Can you work these out from the model? Positions are in its coordinate system, mm. A direction names the side the tool comes from. Round coordinates to 2 decimals unless told otherwise and drop trailing zeros. One line per item, written item: value. Start each with the question number.
(1) Thinking about a two-plate mould opening in X: for faces 1 (the face through (162.11, 20.5, 55.06)), 2 (the face through (149, 21, 77)), which applies, +X half, -X half, draft (parallel to the pull), parting line (faces both ways), or undercut?
(2) I'm going to push flat-ended pins straight in: pin 1 Ø4 at (y, z) = (14.5, 18) entering from -X; pin 2 Ø1 at (y, z) = (22, 49) entering from +X; pin 3 Ø8 at (y, z) = (23, 10.5) entering from +X. Where does each tip first touch, or does it pass through?
(3) If I drill on L1, parallel to Z at x = 140, y = 22.75; L2, parallel to X at y = 14.75, z = 41; L3, parallel to Z at x = 165, y = 20, over which ranges is the centre line in solid material (lowest first)? Write a range as from..to.
(4) I want a section at A-A on z = 32.5. Give the number of separate pieces and of enclosed holes in the cut face, plus the area to 3 significant figures.
(5) On a 3-axis mill with a long thin cutter (end or side, diameter ignored), from which of +Z, -Z, +X, -X, +Y, -Y can I reach the whole of each face in a straight line? I mean faces 3 (the face through (202.885, 11.105, 37.961)), 4 (the face through (153.56, 21.07, 69.94)), 5 (the face through (195.747, 17.752, 38.969)). Say none if no direction works.
Autodesk Inventor part; units mm, degrees
ref_plane "YZ Plane" through (0, 0, 0) normal (1, 0, 0) x (0, 1, 0)
ref_plane "XZ Plane" through (0, 0, 0) normal (0, 1, 0) x (-1, 0, 0)
ref_plane "XY Plane" through (0, 0, 0) normal (0, 0, 1) x (1, 0, 0)
sketch "Sketch2" plane through (0, 0, 0) normal (0, 0, 1) x (1, 0, 0)
  spline S0 degree 5 number of poles 204
  circle A0 centre (79.5137, 4.5678) radius 15.1135
  line L0 (79.5137, 4.5678) -> (79.5137, -15.4763) construction
  line L1 (79.5137, 4.5678) -> (209.6498, 4.5678) construction
  line L2 (319.6498, 0.0573) -> (219.6498, 0.0573) construction
  line L3 (219.6499, 18.7671) -> (219.6499, 18.7671) construction
  line L4 (28.0055, 4.5054) -> (28.0055, -2.4946)
  line L5 (19.6272, 1.0326) -> (319.6498, 0.0573) construction
  line L6 (49.7105, 14.4213) -> (55.6079, 14.4213)
  line L7 (49.7104, -8.4915) -> (55.6078, -8.4915)
  line L8 (28.0055, 4.5054) -> (49.7105, 14.4213)
  line L9 (28.0055, -2.4946) -> (49.7104, -8.4915)
  line L10 (55.6079, 14.4213) -> (55.6079, 20.8729)
  line L11 (55.6078, -8.4915) -> (55.6078, -14.1513)
  line L12 (108.6496, 16.3299) -> (108.6496, -7.1942)
  line L13 (110.8735, -9.1817) -> (193.8736, 0.1678)
  line L14 (195.6498, 2.1552) -> (195.6498, 6.9805)
  arc A1 (108.6496, -7.1942) -> (110.8735, -9.1817) centre (110.6496, -7.1942) ccw
  arc A2 (193.8736, 0.1678) -> (195.6498, 2.1552) centre (193.6498, 2.1552) ccw
  circle A3 centre (209.6498, 0.0573) radius 6.214
  line L15 (108.6496, 18.5678) -> (195.6498, 8.7678)
  circle A4 centre (100.6496, 18.3866) radius 2.5
  circle A5 centre (199.6498, 14.5256) radius 2.5
  spline S1 degree 4 poles (202.7347, 19.3724) (199.838, 19.7251) (195.7649, 20.2061) (190.5032, 20.7952) (184.0435, 21.4697) (179.3239, 21.937) (174.5933, 22.3806) (169.8562, 22.7962) (165.1183, 23.1863) (160.3828, 23.5463) (155.6566, 23.8767) (150.936, 24.1762) (146.2498, 24.4444) (141.5311, 24.676) (136.9019, 24.8782) (132.2312, 25.0296) (127.6189, 25.1375) (123.0371, 25.1982) (118.5028, 25.2125) (112.3622, 25.1677) (107.3995, 25.0507) (103.5849, 24.9119) (100.8865, 24.7866) knots 0 0 0 0 0 0.114234 0.16008 0.206003 0.251978 0.297982 0.343994 0.389991 0.435949 0.481846 0.527693 0.573431 0.619092 0.664656 0.710064 0.755333 0.800383 0.845191 0.889734 1 1 1 1 1
  line L16 (105.191, 21.4637) -> (195.6498, 15.3862)
  arc A6 (100.8865, 24.7866) -> (105.191, 21.4637) centre (100.0416, 19.2427) ccw
  arc A7 (195.6498, 15.3862) -> (202.7347, 19.3724) centre (200.4212, 15.1951) ccw
  point P0 (0, 0)
  point P1 (319.5771, 0.0748)
  point P2 (319.3573, 0.1272)
  point P3 (318.9916, 0.2136)
  point P4 (318.4804, 0.3362)
  point P5 (317.8238, 0.4909)
  point P6 (317.0222, 0.6802)
  point P7 (316.0769, 0.9024)
  point P8 (314.9885, 1.1569)
  point P9 (313.7582, 1.443)
  point P10 (312.3866, 1.7598)
  point P11 (310.8752, 2.1063)
  point P12 (309.2258, 2.4819)
  point P13 (307.4393, 2.8854)
  point P14 (305.5178, 3.3153)
  point P15 (303.4628, 3.7707)
  point P16 (301.2764, 4.2501)
  point P17 (298.9607, 4.7526)
  point P18 (296.5175, 5.2764)
  point P19 (293.9492, 5.8203)
  point P20 (291.2585, 6.3828)
  point P21 (288.4478, 6.9627)
  point P22 (285.5195, 7.5582)
  point P23 (282.4766, 8.1678)
  point P24 (279.3218, 8.79)
  point P25 (276.0584, 9.4236)
  point P26 (272.6891, 10.0668)
  point P27 (269.2175, 10.7178)
  point P28 (265.6469, 11.3757)
  point P29 (261.9803, 12.0381)
  point P30 (258.2219, 12.7041)
  point P31 (254.3747, 13.3722)
  point P32 (250.4426, 14.0403)
  point P33 (246.4295, 14.7072)
  point P34 (242.339, 15.3714)
  point P35 (238.1756, 16.0311)
  point P36 (233.9428, 16.6851)
  point P37 (229.6454, 17.3316)
  point P38 (225.2869, 17.9694)
  point P39 (220.8723, 18.5967)
  point P40 (216.4049, 19.2123)
  point P41 (211.8901, 19.8144)
  point P42 (207.332, 20.4015)
  point P43 (202.7347, 20.9724)
  point P44 (198.1034, 21.5256)
  point P45 (193.4423, 22.0596)
  point P46 (188.7563, 22.5726)
  point P47 (184.0499, 23.0637)
  point P48 (179.3279, 23.5314)
  point P49 (174.5948, 23.9745)
  point P50 (169.8554, 24.3909)
  point P51 (165.1148, 24.7803)
  point P52 (160.3775, 25.1406)
  point P53 (155.6479, 25.4709)
  point P54 (150.9316, 25.7703)
  point P55 (146.233, 26.0373)
  point P56 (141.557, 26.2707)
  point P57 (136.8821, 26.4681)
  point P58 (132.2209, 26.6211)
  point P59 (127.5964, 26.7282)
  point P60 (123.0133, 26.7888)
  point P61 (118.4761, 26.8026)
  point P62 (113.9902, 26.7693)
  point P63 (109.5601, 26.6886)
  point P64 (105.191, 26.5611)
  point P65 (100.8865, 26.3866)
  point P66 (96.6524, 26.1647)
  point P67 (92.4927, 25.8975)
  point P68 (88.412, 25.5858)
  point P69 (84.409, 25.3061)
  point P70 (80.8803, 24.9766)
  point P71 (76.6761, 24.4558)
  point P72 (72.9631, 23.8932)
  point P73 (69.3402, 23.3612)
  point P74 (65.8208, 22.7938)
  point P75 (62.4086, 22.1884)
  point P76 (59.1071, 21.5462)
  point P77 (52.8493, 20.1606)
  point P78 (49.7107, 19.4213)
  point P79 (47.0737, 18.6508)
  point P80 (44.3741, 17.8542)
  point P81 (41.8033, 17.0323)
  point P82 (39.3638, 16.1875)
  point P83 (37.0582, 15.3214)
  point P84 (34.8883, 14.4364)
  point P85 (32.8567, 13.534)
  point P86 (30.9649, 12.6166)
  point P87 (29.2144, 11.686)
  point P88 (27.607, 10.7437)
  point P89 (26.1442, 9.7921)
  point P90 (24.8269, 8.8324)
  point P91 (23.6566, 7.8664)
  point P92 (22.6337, 6.8952)
  point P93 (21.7592, 5.9208)
  point P94 (21.0335, 4.944)
  point P95 (20.4573, 3.966)
  point P96 (20.031, 2.9874)
  point P97 (19.7541, 2.0097)
  point P98 (19.6496, 0.0598)
  point P99 (19.8207, -0.9032)
  point P100 (20.1378, -1.8356)
  point P101 (20.6004, -2.7401)
  point P102 (21.2081, -3.6158)
  point P103 (21.9599, -4.4627)
  point P104 (22.8545, -5.2806)
  point P105 (23.891, -6.069)
  point P106 (25.0682, -6.8277)
  point P107 (26.3845, -7.5561)
  point P108 (27.8383, -8.2539)
  point P109 (29.4283, -8.9211)
  point P110 (31.1522, -9.5571)
  point P111 (33.0086, -10.1613)
  point P112 (34.9949, -10.734)
  point P113 (37.1093, -11.2746)
  point P114 (39.3497, -11.7828)
  point P115 (41.7134, -12.2586)
  point P116 (44.1979, -12.702)
  point P117 (46.8014, -13.1127)
  point P118 (49.7105, -13.4915)
  point P119 (52.3532, -13.8357)
  point P120 (58.3469, -14.4294)
  point P121 (61.5023, -14.678)
  point P122 (64.7591, -14.8953)
  point P123 (68.1149, -15.0813)
  point P124 (71.5661, -15.237)
  point P125 (75.1094, -15.3627)
  point P126 (78.7418, -15.4596)
  point P127 (82.46, -15.528)
  point P128 (86.2607, -15.5691)
  point P129 (90.14, -15.5838)
  point P130 (94.0946, -15.5733)
  point P131 (98.1212, -15.5388)
  point P132 (102.2159, -15.4812)
  point P133 (106.3751, -15.4023)
  point P134 (110.5952, -15.303)
  point P135 (114.872, -15.1845)
  point P136 (119.2022, -15.0489)
  point P137 (123.5813, -14.8971)
  point P138 (128.006, -14.7306)
  point P139 (132.4718, -14.5509)
  point P140 (136.9748, -14.3598)
  point P141 (141.5285, -14.1576)
  point P142 (146.1365, -13.9383)
  point P143 (150.7679, -13.7022)
  point P144 (155.4191, -13.4499)
  point P145 (160.0853, -13.1829)
  point P146 (164.7617, -12.9024)
  point P147 (169.4444, -12.6099)
  point P148 (174.1283, -12.306)
  point P149 (178.8092, -11.9925)
  point P150 (183.4823, -11.67)
  point P151 (188.1434, -11.34)
  point P152 (192.7877, -11.0037)
  point P153 (197.4107, -10.6614)
  point P154 (202.0079, -10.3149)
  point P155 (206.5747, -9.9645)
  point P156 (211.1069, -9.6117)
  point P157 (215.5999, -9.2568)
  point P158 (220.0489, -8.9007)
  point P159 (224.4503, -8.5446)
  point P160 (228.7987, -8.1885)
  point P161 (233.0906, -7.8339)
  point P162 (237.3214, -7.4808)
  point P163 (241.4866, -7.1298)
  point P164 (245.5828, -6.7821)
  point P165 (249.6052, -6.4377)
  point P166 (253.5502, -6.0972)
  point P167 (257.4136, -5.7612)
  point P168 (261.1915, -5.4303)
  point P169 (264.88, -5.1051)
  point P170 (268.4758, -4.7856)
  point P171 (271.9747, -4.4724)
  point P172 (275.3734, -4.1661)
  point P173 (278.6686, -3.867)
  point P174 (281.8564, -3.5757)
  point P175 (284.9344, -3.2925)
  point P176 (287.8984, -3.018)
  point P177 (290.7463, -2.7525)
  point P178 (293.4745, -2.4963)
  point P179 (296.0806, -2.2503)
  point P180 (298.5616, -2.0142)
  point P181 (300.9151, -1.7892)
  point P182 (303.1387, -1.575)
  point P183 (305.23, -1.3728)
  point P184 (307.1866, -1.1823)
  point P185 (309.007, -1.0041)
  point P186 (310.6885, -0.8385)
  point P187 (312.2302, -0.6861)
  point P188 (313.6297, -0.5471)
  point P189 (314.8861, -0.4221)
  point P190 (315.9976, -0.3107)
  point P191 (316.9636, -0.214)
  point P192 (317.7826, -0.1311)
  point P193 (318.4538, -0.0643)
  point P194 (318.9765, -0.0102)
  point P195 (319.3503, 0.027)
  point P196 (319.5743, 0.0497)
  point P197 (28.0055, 1.0054)
  point P198 (108.6496, -9.4322)
  point P199 (195.6498, 0.3678)
  dimension "d37" = 30.227
  dimension "d2" = 300.0001
  dimension "d19" = 110
  dimension "d22" = 100
  dimension "d23" = 7
  dimension "d24" = 5
  dimension "d25" = 5
  dimension "d30" = 28
  dimension "d31" = 8.4
  dimension "d33" = 14
  dimension "d39" = 59.8865
  dimension "d42" = 12.428
  dimension "d43" = 5
  dimension "d44" = 5
  dimension "d49" = 1.6
  dimension "d50" = 1.6
  dimension "d51" = 1.6
  dimension "d52" = 1.6
  dimension "d53" = 1.6
  dimension "d54" = 1.6
  dimension "d55" = 1.6
  dimension "d56" = 1.6
  dimension "d57" = 1.6
  dimension "d58" = 1.6
  dimension "d59" = 1.6
  dimension "d60" = 1.6
  dimension "d61" = 1.6
  dimension "d62" = 1.6
  dimension "d63" = 1.6
  dimension "d64" = 1.6
  dimension "d65" = 1.6
  dimension "d66" = 1.6
  dimension "d67" = 1.6
  dimension "d68" = 1.6
  dimension "d69" = 1.6
  dimension "d70" = 1.6
  dimension "d72" = 1.6
  dimension "d75" = 4
  dimension "d76" = 7
extrude "Extrusion8" add sketch "Sketch2" along normal blind 77 contours A7 L16 A6 S1
sketch "Sketch3" plane through (195.6498, 15.3862, 0) normal (-0.067, -0.9978, 0) x (0.9978, -0.067, 0)
  line L0 (-0.0611, 72) -> (-0.0611, 5)
  line L1 (-0.0611, 5) -> (-22.6844, 38.5)
  line L2 (-22.6844, 38.5) -> (-0.0611, 72)
  line L3 (-67.6844, 38.5829) -> (-45.1844, 72)
  line L4 (-45.1844, 72) -> (-45.1844, 4.8387)
  line L5 (-45.1844, 4.8387) -> (-67.6844, 38.5829)
  line L6 (-45.1844, 72) -> (-22.6844, 38.5)
  line L7 (-45.1844, 4.8387) -> (-22.6844, 38.5)
  line L8 (9.5487, 77) -> (0, 77)
  line L9 (9.5487, 0) -> (0, 0)
  line L10 (-90.3076, 72) -> (-90.0608, 5)
  line L11 (-90.0608, 5) -> (-67.6844, 38.5829)
  line L12 (-90.3076, 72) -> (-67.6844, 38.5829)
  line L13 (-90.0437, 77) -> (-101.2596, 77)
  line L14 (-90.0437, 0) -> (-101.2596, 0)
  line L15 (-90.3076, 72) -> (-0.0611, 72)
  line L16 (-0.0611, 5) -> (-90.0608, 5)
  line L17 (-86.7403, 72) -> (-45.0762, 9.8387)
  line L18 (-86.7403, 5) -> (-45.1844, 67)
  line L19 (-45.1844, 67) -> (-5.985, 5)
  line L20 (-5.985, 72) -> (-45.1844, 10)
  line L21 (-47.5072, 5) -> (-47.5072, 72)
  line L22 (-42.3779, 72) -> (-42.3779, 5)
  point P0 (-194.1783, 0)
  point P1 (-90.6627, 0)
  point P2 (-45.1844, 38.4194)
  point P3 (6.8018, 77)
  point P4 (6.8018, 0)
  point P5 (-95.1802, 77)
  point P6 (-90.6627, 77)
  point P7 (-95.1802, 0)
  point P8 (-27.1653, 38.5)
  point P9 (-64.2867, 38.5)
  point P10 (-24.9925, 41.9366)
  point P11 (-45.2266, 49)
  point P12 (-66.0095, 41.0704)
  point P13 (-45.2288, 49)
  point P14 (-24.9871, 35.0549)
  point P15 (-65.9622, 36.0001)
  point P16 (-42.3779, 9.0373)
  point P17 (-42.3779, 62.5611)
  point P18 (-42.3779, 14.4389)
  point P19 (-42.3779, 67.8215)
  point P20 (-47.5072, 68.5501)
  point P21 (-47.5072, 8.3224)
  point P22 (-47.5072, 13.4656)
  point P23 (-47.5072, 63.5344)
  dimension "d81" = 22.5
  dimension "d82" = 22.5
  dimension "d83" = 5
  dimension "d84" = 5
  dimension "d85" = 22.5
  dimension "d86" = 5
  dimension "d87" = 5
  dimension "d90" = 5
  dimension "d91" = 5
extrude "Extrusion9" cut sketch "Sketch3" against normal blind 10 contours L0 L1 L2 | L20 L6 L22 L15 | L16 L22 L7 L19 | L20 L22 L19 | L3 L17 L15 L21 | L21 L17 L18 | L11 L10 L12 | L21 L16 L18 L5
properties part number "2414 basic aerofoil" material "Plywood, Finish"
Established:
1. face 1: undercut
1. face 2: draft
2. pin 1: x = 95.15
2. pin 2: x = 180.76
2. pin 3: x = 203.31
3. L1: 0..5, 21.09..26.16, 50.84..55.91, 72..77
3. L2: 96.69..103.4, 195.67..197.16, 202.14..205.18
3. L3: 0..5, 26.22..32.61, 44.39..50.72, 72..77
4. separate pieces: 7
4. enclosed holes: 2
4. area: 258 mm2
5. face 3: +Z, -Z
5. face 4: -Y
5. face 5: +Y
